Input: part model. Units: mm. Frame: model coordinates. A direction names the side the tool comes from. Give positions to 0.01 mm unless a question says otherwise; leave off trailing zeros. Write each loop counter-clockwise with the first axis right and the second up, starting at its lowest first coordinate (ties: lowest second). Pieces come first, ordered by that corner, then holes. Notation, with made-up numbers: M 81.5,61.25 L 99.5,61.25 A23 cw 99.5,77.25 Z; hole C -23.75,-15.5 d8. An arc over 180 degrees is marked long. Use CSV: the item, a comma, the result in double quotes. Start each with the question number.
from build123d import *

# Parameters (mm, degrees)
PAD_DEPTH            = 18.2
SKETCH003_W          = 19.45
SKETCH003_H          = 39
POCKET_DEPTH         = 14.001
POCKET001_DEPTH      = 5.101
POCKET002_DEPTH      = 57.6
SKETCH011_W          = 5.3
SKETCH011_H          = 2.3
POCKET004_DEPTH      = 5
PAD005_DEPTH         = 10
PAD005_DEPTH_BACK    = 2.1
SKETCH014_W          = 10
SKETCH014_H          = 2.1
PAD006_DEPTH         = 5
CHAMFER001_SIZE      = 0.5
POCKET005_DEPTH      = 3
POCKET006_DEPTH      = 100
POCKET006_DEPTH_BACK = 100
FILLET001_R          = 1
SKETCH017_W          = 4
SKETCH017_H          = 1.2
SKETCH017_W_2        = 3.5
SKETCH017_H_2        = 4.5
SKETCH017_H_3        = 3.3
PAD008_DEPTH         = 2
CHAMFER_SIZE         = 0.9


with BuildPart() as body:
    # Sketch002 → Pad (new body)
    with BuildSketch(Plane.XY.offset(13.1)):
        Polygon((9, 0), (9, 1.3), (-23.5, 1.3), (-23.5, -1.7), (-29.55, -1.7), (-29.55, -65.7), (-10.45, -65.7), (-10.45, -39), (9, -39), align=None)
    extrude(amount=-PAD_DEPTH)

    # Sketch003 → Pocket (cut, through all)
    with BuildSketch(Plane.XY.offset(8.9)):
        with Locations((-0.725, -19.5)):
            Rectangle(SKETCH003_W, SKETCH003_H)
    extrude(amount=-POCKET_DEPTH, mode=Mode.SUBTRACT)

    # Sketch007 → Pocket001 (cut, through all)
    with BuildSketch(Plane.XY):
        Polygon((21.5, 0), (-21.8, 0), (-21.8, -3.4), (-27.85, -3.4), (-27.85, -61), (-21.8, -61), (-21.8, -68.9), (21.5, -68.9), align=None)
    extrude(amount=-POCKET001_DEPTH, mode=Mode.SUBTRACT)

    # Sketch008 → Pocket002 (cut)
    with BuildSketch(Plane.XZ.offset(3.4)):
        with BuildLine():
            ThreePointArc((-12.786305, 8.9), (-14.580794, 10.759754), (-16.9, 11.9))
            Line((-21.1, 11.9), (-16.9, 11.9))
            ThreePointArc((-21.1, 11.9), (-23.419206, 10.759754), (-25.213695, 8.9))
            Line((-25.213695, 8.9), (-27.55, 8.9))
            Line((-27.55, 8.9), (-27.55, -3.6))
            Line((-27.55, -3.6), (-10.45, -3.6))
            Line((-10.45, 8.9), (-10.45, -3.6))
            Line((-12.786305, 8.9), (-10.45, 8.9))
        make_face()
    extrude(amount=POCKET002_DEPTH, mode=Mode.SUBTRACT)

    # Sketch011 → Pocket004 (cut)
    with BuildSketch(Plane.XZ):
        with Locations((0, -3.95)):
            Rectangle(SKETCH011_W, SKETCH011_H)
        with BuildLine():
            Line((-4.65, 3.35), (-4.65, 5.65))
            ThreePointArc((-4.15, 6.15), (-4.503553, 6.003553), (-4.65, 5.65))
            Line((-4.15, 6.15), (4.15, 6.15))
            ThreePointArc((4.65, 5.65), (4.503553, 6.003553), (4.15, 6.15))
            Line((4.65, 5.65), (4.65, 3.35))
            ThreePointArc((4.15, 2.85), (4.503553, 2.996447), (4.65, 3.35))
            Line((4.15, 2.85), (-4.15, 2.85))
            ThreePointArc((-4.65, 3.35), (-4.503553, 2.996447), (-4.15, 2.85))
        make_face()
    extrude(amount=-POCKET004_DEPTH, mode=Mode.SUBTRACT)

    # Sketch012 → Pad005 (join, two sides)
    with BuildSketch(Plane.XY) as pad005_sk:
        Polygon((1.1, -38), (0.55, -37.047372), (-0.55, -37.047372), (-1.1, -38), (-0.55, -38.952628), (0.55, -38.952628), align=None)
    extrude(amount=PAD005_DEPTH)
    extrude(pad005_sk.sketch, amount=-PAD005_DEPTH_BACK)

    # Sketch014 → Pad006 (join)
    with BuildSketch(Plane.XY.offset(4)):
        with Locations((0, -38)):
            Rectangle(SKETCH014_W, SKETCH014_H)
    extrude(amount=PAD006_DEPTH)

    # Chamfer001
    chamfer001_edges = [body.edges().sort_by_distance(p)[0] for p in [
        (0.825, -37.523686, -2.1),
        (0, -37.047372, -2.1),
        (-0.825, -37.523686, -2.1),
        (-0.825, -38.476314, -2.1),
        (0, -38.952628, -2.1),
        (0.825, -38.476314, -2.1),
    ]]
    chamfer(chamfer001_edges, length=CHAMFER001_SIZE)

    # Sketch013 → Pocket005 (cut)
    with BuildSketch(Plane.XY):
        with BuildLine():
            Line((-20.25, -62.3), (-20.25, -63.1))
            ThreePointArc((-20.25, -63.1), (-19.883883, -63.983883), (-19, -64.35))
            Line((-16, -64.35), (-19, -64.35))
            ThreePointArc((-16, -64.35), (-15.116117, -63.983883), (-14.75, -63.1))
            Line((-14.75, -1.3), (-14.75, -63.1))
            ThreePointArc((-14.75, -1.3), (-15.116117, -0.416117), (-16, -0.05))
            Line((-19, -0.05), (-16, -0.05))
            ThreePointArc((-19, -0.05), (-19.883883, -0.416117), (-20.25, -1.3))
            Line((-20.25, -1.3), (-20.25, -2.1))
            Line((-20.25, -2.1), (-20.25, -62.3))
        make_face()
    extrude(amount=POCKET005_DEPTH, mode=Mode.SUBTRACT)

    # Sketch016 → Pocket006 (cut, two sides)
    with BuildSketch(Plane.XZ) as pocket006_sk:
        with BuildLine():
            ThreePointArc((-21.55, 13.1), (-27.206854, 10.756854), (-29.55, 5.1))
            Line((-29.55, 5.1), (-32.473244, 5.1))
            Line((-32.473244, 5.1), (-32.473244, 16.532589))
            Line((-32.473244, 16.532589), (-21.55, 16.532589))
            Line((-21.55, 16.532589), (-21.55, 13.1))
        make_face()
    extrude(amount=POCKET006_DEPTH, mode=Mode.SUBTRACT)
    extrude(pocket006_sk.sketch, amount=-POCKET006_DEPTH_BACK, mode=Mode.SUBTRACT)

    # Fillet001
    fillet001_edges = [body.edges().sort_by_distance(p)[0] for p in [
        (9, -19.5, 13.1),
        (-0.725, -39, 13.1),
        (-10.45, -52.35, 13.1),
        (-16, -65.7, 13.1),
        (-21.55, -32.2, 13.1),
        (-6.275, 1.3, 13.1),
        (9, 0.65, 13.1),
        (-22.532436, 1.3, 13.039447),
        (-23.5, 1.3, 3.879352),
        (-23.5, -0.2, 12.858705),
        (-23.5, -1.7, 3.879352),
        (-29.55, -1.7, 0),
        (-27.858724, -1.7, 10.01935),
        (-29.55, -65.7, 0),
        (-27.206854, -65.7, 10.756854),
        (-10.45, -65.7, 6.55),
        (-10.45, -39, 11),
        (9, -39, 11),
        (9, 1.3, 4),
    ]]
    fillet(fillet001_edges, radius=FILLET001_R)

    # Sketch017 → Pad008 (join)
    with BuildSketch(Plane.XY.offset(-1.6)):
        with Locations((7, -0.6)):
            Rectangle(SKETCH017_W, SKETCH017_H)
        with Locations((-21.55, -63.45)):
            Rectangle(SKETCH017_W_2, SKETCH017_H_2)
        with Locations((-21.55, -1.65)):
            Rectangle(SKETCH017_W_2, SKETCH017_H_3)
    extrude(amount=-PAD008_DEPTH)

    # Chamfer
    chamfer_edges = [body.edges().sort_by_distance(p)[0] for p in [
        (-19.8, -1.65, -1.6),
        (-19.8, -63.45, -1.6),
    ]]
    chamfer(chamfer_edges, length=CHAMFER_SIZE)


with BuildPart() as part_mirroring:
    # Part__Mirroring: instance of Body
    add(body.part.mirror(Plane(origin=(-10.604568, -32.200001, 0), x_dir=(0, 1, 0), z_dir=(0, 0, 1))))


with BuildPart() as part_mirroring_1:
    # Part__Mirroring placement: moved
    add(part_mirroring.part.moved(Location((0, 0, -15))))


solid = part_mirroring_1.part
Q1. Section C-C, the plane y = -7.5. Return the cut outline in (x, z).
Q2. Section B-B, the plane y = -43.5. Return the cut outline in (x, z).
Q3. Section A-A, the plane x = -3.5. Return the cut outline in (y, z).
Q4. Set-up query: faces 5 (the cylindrical face through (-23.39, -31.8, -25.78)), 6 (the flat face through (-20.25, -62, -16)), 7 (the flat face through (-14.9, -64.4, -15)). Return all of +Z, -Z, +X, -X, +Y, -Y with unobstructed straight access to the full face (end or side cutting, diameter ignored); none if empty.
Q5. Pull-direction query (X, two-part tool) for faces 1 (the flat face through (7, -1.2, -12)), 2 (the cylindrical face through (-19.874, -0.406, -16.479)), 3 (the flat face through (0, 1, -17.85)), 4 (the flat face through (-29.55, -33, -15)); classes: released by +X, released by -X, zero draft, split by the parting line, or undercut.
Q6. First-contact query: pin 1 Ø4 at (y, z) = (-57.5, -23.5) entering from -X; pin 2 Ø1 at (y, z) = (-2, -16.5) entering from -X; pin 3 Ø1.1 at (y, z) = (-62, -16.5) entering from +X. Flat tips, straight axial feed; report the tip coordinate or a pass-through.
Q7. Material intervals for L1, parallel to Y at x = -22.5, z = -13.25; L2, parallel to Y at x = -2, z = -26; L3, parallel to Z at x = -2.5, y = -18, sorted ascending. Write a range as [from, to].
Check result:
1,outline,"M -29.55,-20.1 A8 ccw -21.55,-28.1 L 8,-28.1 A1 ccw 9,-27.1 L 9,-23.9 L -12.79,-23.9 A7.5 cw -16.9,-26.9 L -21.1,-26.9 A7.5 cw -25.21,-23.9 L -27.55,-23.9 L -27.55,-15 L -27.85,-15 L -27.85,-9.9 L -29.55,-9.9 Z"
2,outline,"M -29.55,-20.1 A8 ccw -21.55,-28.1 L -11.45,-28.1 A1 ccw -10.45,-27.1 L -10.45,-23.9 L -12.79,-23.9 A7.5 cw -16.9,-26.9 L -21.1,-26.9 A7.5 cw -25.21,-23.9 L -27.55,-23.9 L -27.55,-15 L -27.85,-15 L -27.85,-9.9 L -29.55,-9.9 Z"
3,outline,"M -39.05,-24 L -39,-24 L -39,-27.1 A1 ccw -38,-28.1 L 0.3,-28.1 A1 ccw 1.3,-27.1 L 1.3,-21.15 L 0,-21.15 L 0,-23.9 L -36.95,-23.9 L -36.95,-19 L -39.05,-19 Z; M 0,-17.85 L 1.3,-17.85 L 1.3,-9.9 L 0,-9.9 Z"
4,face 5,"+Z"
4,face 6,"none"
4,face 7,"+X, -Y"
5,face 1,"zero draft"
5,face 2,"undercut"
5,face 3,"undercut"
5,face 4,"released by -X"
6,pin 1,"stops at x = -29.43"
6,pin 2,"stops at x = -29.53"
6,pin 3,"stops at x = -10.45"
7,L1,"y = [-65.7, -61], [-3.4, 1.3]"
7,L2,"y = [-39, 1.3]"
7,L3,"z = [-28.1, -23.9]"
